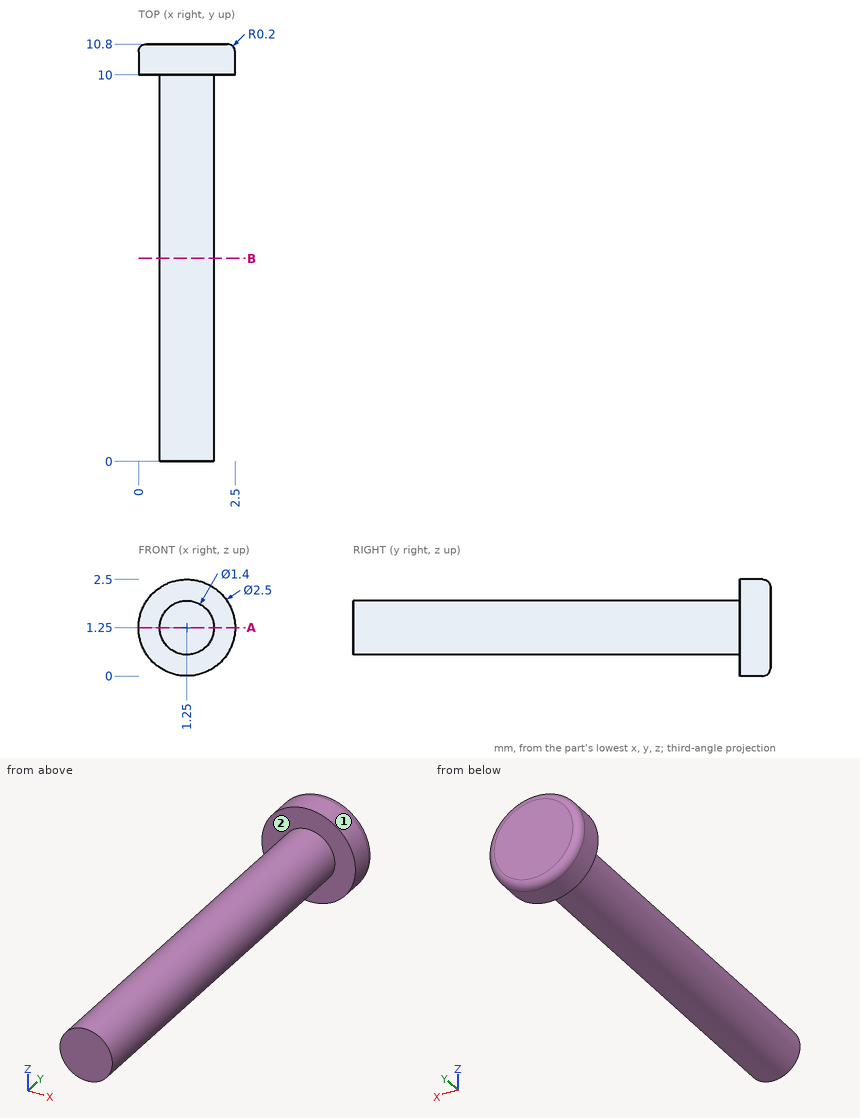
The figure shows three views and two pictorial views of one solid part (mm, origin at its lowest corner). Answer the questions. A direction names the side the tool comes from. Coordinates: 2 decimals unless noted, no trailing zeros. Loops run counter-clockwise (first coordinate to the right, second up) from the corner with the lowest first, then second, coordinate; pieces in that order, holes last. Notation, with made-up numbers: (-27, -11) -> (-16, -11) arc R24 cw to (-16, 24) -> close; hole circle Ø8 at (55, 51). An arc over 180 degrees is marked (long way). Return JSON: item names as keys, results as strings. Group by question number.
(1) A cutting plane is placed at A-A on z = 1.25. Write down the section's boundary in (x, y).
(2) Given pin 1 Ø1.5 at (x, y) = (1.5, 1.5) entering from -Z, flat-ended and moving along its own axis, determine where the tip first touches the part or whether it passes through.
(3) A cutting plane is placed at B-B on y = 5.25. Write down the section's boundary in (x, z).
(4) Which of the six approach directions +Z, -Z, +X, -X, +Y, -Y give full straight-line access (tool end or side, diameter ignored) to the marked faces 1 and 2?
(5) Find the intervals of material crossed by probe 1 along Y at (x, z) = (2.15, 1.3); probe 2 along X at (y, z) = (2, 1.2); probe 3 along X at (y, z) = (8.75, 1.8), in increasing order. Write a range as from..to.
The answers:
{
 "1": {"outline": "(0, 10) -> (0.55, 10) -> (0.55, 0) -> (1.95, 0) -> (1.95, 10) -> (2.5, 10) -> (2.5, 10.6) arc R0.2 ccw to (2.3, 10.8) -> (0.2, 10.8) arc R0.2 ccw to (0, 10.6) -> close"},
 "2": {"pin 1": "stops at z = 0.55"},
 "3": {"outline": "circle Ø1.4 at (1.25, 1.25)"},
 "4": {"face 1": "+Y, -Y", "face 2": "-Y"},
 "5": {"probe 1": "y = 10..10.8", "probe 2": "x = 0.55..1.95", "probe 3": "x = 0.82..1.68"}
}
